Drawing for the job (mm, zero at the part's lowest x, y, z). A direction names the side the tool comes from. Give positions to 0.01 mm unless a question says otherwise; leave off trailing zeros. Order: outer loops, then holes, each group sorted by start corner. A loop starts at its lowest first (then second) coordinate and runs counter-clockwise, first axis right, second up. Notation, with made-up numbers: (54.5, 40.5) - (101.5, 40.5) arc R24 cw to (101.5, 71.5) - close; hole circle Ø9 at (-34, 1.25). An arc over 180 degrees is marked (long way). Use a Markdown table: item, result. Add a question column.
(1) Mould opens along Y. For the marked faces 1, 2, 3 and 4 say: +Y half, -Y half, draft (parallel to the pull), parting line (faces both ways), or undercut.
(2) Wall check: line 1 (Z direction, x = 31, y = 66.5); line 2 (Z direction, x = 43.5, y = 54.5); line 3 (Z direction, x = 50.5, y = 27). Give the ranges that are in metal, low to high.
(3) Slice it at B-B (z = 79). Write the cut outline in (x, y).
(4) Flat gauge pins, fed straight in: pin 1 (22 mm diameter, centred on x = 26.5, z = 79.5, fed in from +Y); pin 2 (3 mm diameter, centred on y = 51.5, z = 62.5, fed in from +X); pin 3 (6 mm diameter, centred on y = 68.5, z = 67.5, fed in from -X). Where does each tip first touch, or does it go through?
(5) Which spindle directions (+Z, -Z, +X, -X, +Y, -Y) get a long thin tool onto all of the face, cutting with end or side? Do the marked faces 5, 6, 7, 8 and 9. Say none if no direction does.
(6) Slice it at A-A (y = 25). Write the cut outline in (x, z).
(7) Slice it at C-C (x = 16.5). Write the cut outline in (y, z), then the cut area to 3 significant figures.
(8) Slice it at D-D (y = 12.5). Write the cut outline in (x, z), then the cut area to 3 significant figures.
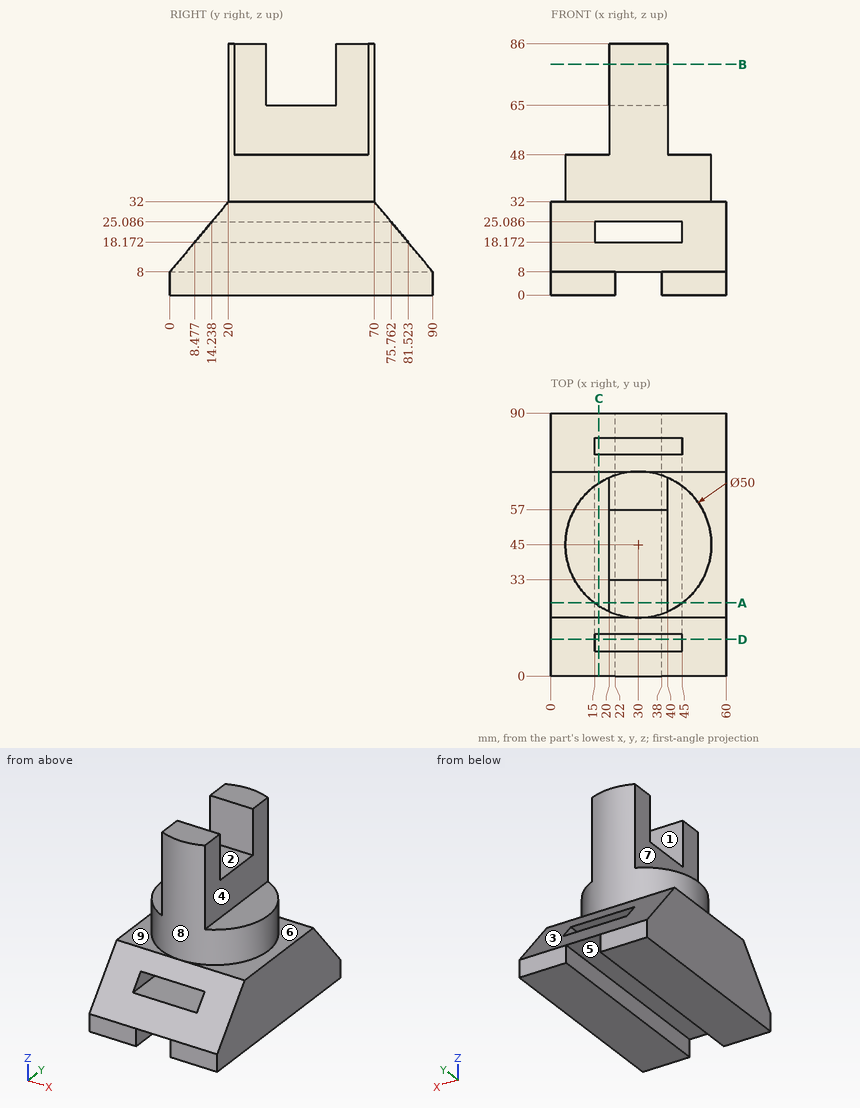
Solution:
| question | item | result |
|---|---|---|
| 1 | face 1 | undercut |
| 1 | face 2 | undercut |
| 1 | face 3 | +Y half |
| 1 | face 4 | draft |
| 2 | line 1 | 8 to 18.17, 25.09 to 86 |
| 2 | line 2 | 0 to 18.17, 25.09 to 48 |
| 2 | line 3 | 0 to 32 |
| 3 | outline | (20, 22.09) arc R25 ccw to (40, 22.09) - (40, 33) - (20, 33) - close; (20, 57) - (40, 57) - (40, 67.91) arc R25 ccw to (20, 67.91) - close |
| 4 | pin 1 | y = 70 |
| 4 | pin 2 | x = 40 |
| 4 | pin 3 | x = 20 |
| 5 | face 5 | -Z, +Y, -Y |
| 5 | face 6 | +Z, +X |
| 5 | face 7 | +Z, -X, +Y, -Y |
| 5 | face 8 | +Z |
| 5 | face 9 | +Z, -X |
| 6 | outline | (0, 0) - (22, 0) - (22, 8) - (38, 8) - (38, 0) - (60, 0) - (60, 32) - (45, 32) - (45, 48) - (40, 48) - (40, 86) - (20, 86) - (20, 48) - (15, 48) - (15, 32) - (0, 32) - close; hole (15, 18.17) - (45, 18.17) - (45, 25.09) - (15, 25.09) - close |
| 7 | outline | (0, 0) - (90, 0) - (90, 8) - (81.52, 18.17) - (8.48, 18.17) - (0, 8) - close; (14.24, 25.09) - (75.76, 25.09) - (70, 32) - (66.04, 32) - (66.04, 48) - (23.96, 48) - (23.96, 32) - (20, 32) - close |
| 7 | area | 2,610 mm2 |
| 8 | outline | (0, 0) - (22, 0) - (22, 8) - (38, 8) - (38, 0) - (60, 0) - (60, 23) - (45, 23) - (45, 18.17) - (15, 18.17) - (15, 23) - (0, 23) - close |
| 8 | area | 1,110 mm2 |
